Part model, mm, in its own coordinate system. A direction names the side the tool comes from. Round coordinates to 2 decimals unless told otherwise and drop trailing zeros. Loops run counter-clockwise (first coordinate to the right, second up) from the corner with the lowest first, then second, coordinate; pieces in that order, holes last.
from build123d import *

# Parameters (mm, degrees)
SKETCH1_R         = 49.1363
EXTRUDE1_DEPTH    = 85.09
SKETCH5_R         = 3.96875
EXTRUDE5_DEPTH    = 26.67
SKETCH2_OUTSIDE_W = 132.864
SKETCH2_OUTSIDE_H = 132.864
SKETCH2_OUTSIDE_R = 14.2875
EXTRUDE2_DEPTH    = 28.956
SKETCH3_OUTSIDE_W = 132.864
SKETCH3_OUTSIDE_H = 132.864
SKETCH3_OUTSIDE_R = 23.9268
EXTRUDE3_DEPTH    = 12.7762
SKETCH4_OUTSIDE_W = 132.864
SKETCH4_OUTSIDE_H = 132.864
SKETCH4_OUTSIDE_R = 46.228
EXTRUDE4_DEPTH    = 32.9057
SKETCH6_R         = 42.3545
SKETCH6_R_2       = 23.9268
EXTRUDE8_DEPTH    = 23.368
SKETCH7_R         = 19.177
EXTRUDE9_DEPTH    = 50.8
SKETCH8_OUTSIDE_W = 132.864
SKETCH8_OUTSIDE_H = 132.864
SKETCH8_OUTSIDE_R = 41.7576
EXTRUDE10_DEPTH   = 7.112
CHAMFER1_SIZE     = 1.27
CHAMFER1_SIZE2    = 8.636


with BuildPart() as part:
    # Sketch1 → Extrude1 (new body)
    with BuildSketch(Plane.XY):
        Circle(SKETCH1_R)
    extrude(amount=EXTRUDE1_DEPTH)

    # Sketch5 → Extrude5 (cut)
    with BuildSketch(Plane.XY.offset(85.09)):
        Circle(SKETCH5_R)
    extrude(amount=-EXTRUDE5_DEPTH, mode=Mode.SUBTRACT)

    # Sketch2 outside → Extrude2 (cut)
    with BuildSketch(Plane.XY.offset(85.09)):
        Rectangle(SKETCH2_OUTSIDE_W, SKETCH2_OUTSIDE_H)
        Circle(SKETCH2_OUTSIDE_R, mode=Mode.SUBTRACT)
    extrude(amount=-EXTRUDE2_DEPTH, mode=Mode.SUBTRACT)

    # Sketch3 outside → Extrude3 (cut)
    with BuildSketch(Plane.XY.offset(56.134)):
        Rectangle(SKETCH3_OUTSIDE_W, SKETCH3_OUTSIDE_H)
        Circle(SKETCH3_OUTSIDE_R, mode=Mode.SUBTRACT)
    extrude(amount=-EXTRUDE3_DEPTH, mode=Mode.SUBTRACT)

    # Sketch4 outside → Extrude4 (cut)
    with BuildSketch(Plane(origin=(0, 0, 0), x_dir=(-1, 0, 0), z_dir=(0, 0, -1))):
        Rectangle(SKETCH4_OUTSIDE_W, SKETCH4_OUTSIDE_H)
        Circle(SKETCH4_OUTSIDE_R, mode=Mode.SUBTRACT)
    extrude(amount=-EXTRUDE4_DEPTH, mode=Mode.SUBTRACT)

    # Sketch6 → Extrude8 (cut)
    with BuildSketch(Plane.XY.offset(43.3578)):
        Circle(SKETCH6_R)
        Circle(SKETCH6_R_2, mode=Mode.SUBTRACT)
    extrude(amount=-EXTRUDE8_DEPTH, mode=Mode.SUBTRACT)

    # Sketch7 → Extrude9 (cut)
    with BuildSketch(Plane(origin=(0, 0, 0), x_dir=(-1, 0, 0), z_dir=(0, 0, -1))):
        Circle(SKETCH7_R)
    extrude(amount=-EXTRUDE9_DEPTH, mode=Mode.SUBTRACT)

    # Sketch8 outside → Extrude10 (cut)
    with BuildSketch(Plane(origin=(0, 0, 0), x_dir=(-1, 0, 0), z_dir=(0, 0, -1))):
        Rectangle(SKETCH8_OUTSIDE_W, SKETCH8_OUTSIDE_H)
        Circle(SKETCH8_OUTSIDE_R, mode=Mode.SUBTRACT)
    extrude(amount=-EXTRUDE10_DEPTH, mode=Mode.SUBTRACT)

    # Chamfer1
    chamfer1_edges = [part.edges().sort_by_distance(p)[0] for p in [
        (-42.3545, 0, 43.3578),
    ]]
    chamfer1_side = [part.faces().sort_by_distance(p)[0] for p in [
        (-47.746515563, 0, 43.3578),
    ]]
    chamfer(chamfer1_edges, length=CHAMFER1_SIZE, length2=CHAMFER1_SIZE2, reference=chamfer1_side[0])


solid = part.part
1) Drop flat-ended pins along their axis: pin 1 Ø6 at (x, z) = (-17, 28) entering from +Y; pin 2 Ø2 at (x, z) = (4, 59.5) entering from +Y; pin 3 Ø4 at (x, y) = (-0.5, -0.5) entering from +Z. Give the stop position or say it passes through.
Values:
pin 1: stops at y = 44.06
pin 2: stops at y = 13.97
pin 3: stops at z = 58.42
2) Slice it at D-D, the plane z = 10.5. Give the cut face in (x, y).
Values:
outline: circle Ø92.46 at (0, 0); hole circle Ø38.35 at (0, 0)
3) Mould opens along X. For faces 1 (the face through (34.5, -23.8, 7.112)), 2 (the face through (-5.514, 41.994, 27.459)), 3 (the face through (-38.573, -15.993, 3.506)) say: released by +X, released by -X, zero draft, split by the parting line, or undercut.
Values:
face 1: zero draft
face 2: undercut
face 3: split by the parting line
4) Slice it at C-C, the plane z = 38.5. Give the cut face in (x, y).
Values:
outline: circle Ø98.27 at (0, 0); circle Ø47.85 at (0, 0); hole circle Ø85.82 at (0, 0); hole circle Ø38.35 at (0, 0)
5) Tool access for faces 4 (the face through (-33, 33, 32.906)), 5 (the face through (10.3, -10.3, 56.134)), 6 (the face through (9, -18, 0)): list every direction of +Z, -Z, +X, -X, +Y, -Y with a clear straight run to the whole face (end or side of a thin tool).
Values:
face 4: -Z
face 5: +Z
face 6: -Z, +X, -X, +Y, -Y
6) Wall check: line 1 along Y through (x, z) = (0, 23.75); line 2 along Y through (x, z) = (-17.5, 40); line 3 along Y through (x, z) = (0, 11). Give the ranges that are in metal, low to high.
Values:
line 1: y = -46.23 to -42.35, -23.93 to -19.18, 19.18 to 23.93, 42.35 to 46.23
line 2: y = -45.91 to -39.42, -16.32 to -7.84, 7.84 to 16.32, 39.42 to 45.91
line 3: y = -46.23 to -19.18, 19.18 to 46.23
